Autodesk Inventor part; units mm, degrees
ref_plane "YZ Plane" through (0, 0, 0) normal (1, 0, 0) x (0, 1, 0)
ref_plane "XZ Plane" through (0, 0, 0) normal (0, 1, 0) x (-1, 0, 0)
ref_plane "XY Plane" through (0, 0, 0) normal (0, 0, 1) x (1, 0, 0)
sketch "Sketch1" plane through (0, 0, 0) normal (0, 1, 0) x (-1, 0, 0)
  line L0 (0, 0) -> (36, 0)
  line L1 (36, 0) -> (36, -24)
  line L2 (36, -24) -> (0, -24)
  line L3 (0, -24) -> (0, 0)
  dimension "d0" = 36
  dimension "d1" = 24
extrude "Extrusion1" add sketch "Sketch1" along normal blind 3
sketch "Sketch2" plane through (0, 3, 0) normal (0, 1, 0) x (1, 0, 0)
  circle A0 centre (-6, 12) radius 2.125
  point P0 (0, 0)
  dimension "d4" = 4.25
extrude "Extrusion2" cut sketch "Sketch2" against normal through all
pattern_linear "Rectangular Pattern1" count 3 spacing 12 along (-1, 0, 0) count 3 spacing 6 along (0, 0, 1) of "Extrusion2" second direction both ways yes
sketch "Sketch3" plane through (0, 0, 0) normal (1, 0, 0) x (0, 0, -1)
  line L0 (0, 0) -> (24, 0)
  line L1 (24, 0) -> (24, 3)
  line L2 (24, 3) -> (0, 3)
  line L3 (0, 3) -> (0, 0)
extrude "Extrusion3" add sketch "Sketch3" along normal blind 25
sketch "Sketch4" plane through (0, 3, 0) normal (0, 1, 0) x (1, 0, 0)
  line L0 (-36, 24) -> (25, 24)
  line L1 (25, 0) -> (22, 0)
  line L2 (22, 0) -> (22, 24)
  line L3 (22, 24) -> (25, 24)
  line L4 (25, 24) -> (25, 0)
  point P0 (0, 0)
  dimension "d15" = 3
extrude "Extrusion4" add sketch "Sketch4" along normal blind 57
sketch "Sketch5" plane through (22, 3, -24) normal (-1, 0, 0) x (0, 0, 1)
  line L0 (24, 57) -> (24, 33)
  line L1 (24, -3) -> (24, 57)
  line L2 (0, -3) -> (0, 57)
  line L3 (24, 33) -> (0, 33)
  line L4 (0, 33) -> (0, 30)
  line L5 (0, 30) -> (24, 30)
  line L6 (24, 30) -> (24, 33)
  dimension "d18" = 24
  dimension "d19" = 3
extrude "Extrusion5" add sketch "Sketch5" along normal blind 7
sketch "Sketch6" plane through (22, 36, 0) normal (0, 1, 0) x (1, 0, 0)
  line L0 (-7, 0) -> (-5, 0)
  line L1 (-5, 0) -> (-5, 2)
  line L2 (-5, 2) -> (-7, 2)
  line L3 (-7, 2) -> (-7, 0)
  line L4 (-7, 24) -> (-5, 24)
  line L5 (-5, 24) -> (-5, 22)
  line L6 (-5, 22) -> (-7, 22)
  line L7 (-7, 22) -> (-7, 24)
  point P0 (-22, 0)
  dimension "d22" = 2
  dimension "d23" = 2
  dimension "d24" = 2
  dimension "d25" = 2
extrude "Extrusion6" add sketch "Sketch6" along normal blind 24
sketch "Sketch7" plane through (25, 0, -24) normal (0, 0, -1) x (-1, 0, 0)
  line L0 (0, 60) -> (10, 60)
  line L1 (10, 60) -> (10, 33)
  line L2 (10, 33) -> (0, 33)
  line L3 (0, 33) -> (0, 60)
  point P0 (25, 0)
extrude "Extrusion7" add sketch "Sketch7" along normal blind 3
sketch "Sketch8" plane through (-36, 0, 0) normal (0, 0, 1) x (1, 0, 0)
  line L0 (51, 33) -> (61, 33)
  line L1 (61, 33) -> (61, 60)
  line L2 (61, 60) -> (51, 60)
  line L3 (51, 60) -> (51, 33)
  point P0 (36, 0)
extrude "Extrusion8" add sketch "Sketch8" along normal blind 3
sketch "Sketch9" plane through (-36, 0, 0) normal (0, 0, 1) x (1, 0, 0)
  line L0 (0, 0) -> (61, 0)
  line L1 (61, 0) -> (61, 33)
  line L2 (61, 33) -> (0, 33)
  line L3 (0, 33) -> (0, 0)
  point P0 (36, 0)
sketch "Sketch10" plane through (0, 60, 0) normal (0, 1, 0) x (1, 0, 0)
  line L0 (22, 0) -> (22, -1)
  line L1 (22, 24) -> (22, 25)
  line L2 (22, -1) -> (17, -1)
  line L3 (17, -1) -> (17, 25)
  line L4 (17, 25) -> (22, 25)
  line L5 (22, 25) -> (22, -1)
  point P0 (0, 0)
  dimension "d34" = 1
  dimension "d35" = 1
extrude "Extrusion10" cut sketch "Sketch10" against normal through all
sketch "Sketch11" plane through (-36, 0, -24) normal (0, 0, -1) x (-1, 0, 0)
  line L0 (-58, 33) -> (-58, 0)
  line L1 (-53, 0) -> (-58, 0)
  line L2 (-58, 0) -> (-58, 3)
  line L3 (-58, 3) -> (-53, 3)
  line L4 (-53, 3) -> (-53, 0)
  point P0 (-36, 0)
extrude "Extrusion11" add sketch "Sketch11" against normal blind 24
sketch "Sketch12" plane through (-36, 0, -24) normal (0, 0, -1) x (-1, 0, 0)
  line L0 (-36, 0) -> (0, 20.7846)
  line L1 (-36, 0) -> (5.5692, 0) construction
  line L2 (0, 20.7846) -> (-1.5, 23.3827)
  line L3 (-1.5, 23.3827) -> (-37.5, 2.5981)
  line L4 (-37.5, 2.5981) -> (-36, 0)
  dimension "d47" = 30
  dimension "d48" = 3
ref_plane "Work Plane1" through (0.3404, 3, 0) normal (0.2240446, 0.9745789, 0) x (0.9745789, -0.2240446, 0)
extrude "Extrusion14" add sketch "Sketch12" against normal blind 24
sketch "Sketch15" plane through (-36, 0, -24) normal (0, 0, -1) x (-1, 0, 0)
  line L0 (0, 3) -> (-30.8038, 3)
  line L1 (0, 3) -> (-30.8038, 3)
  line L2 (-30.8038, 3) -> (-36, 0)
  line L3 (-36, 0) -> (0, 0)
  line L4 (0, 0) -> (-61, 0)
  line L5 (0, 0) -> (0, 3)
extrude "Extrusion15" cut sketch "Sketch15" against normal through all
sketch "Sketch16" plane through (0.8038, 3, 0) normal (0.5, 0.8660254, 0) x (0.8660254, -0.5, 0)
  line L0 (-40.7654, 24) -> (-40.7654, 0)
  line L1 (-40.7654, 12) -> (-34.7654, 12)
  circle A0 centre (-34.7654, 12) radius 2.125
  point P0 (0.8038, 0)
  dimension "d53" = 6
  dimension "d54" = 4.25
extrude "Extrusion16" cut sketch "Sketch16" against normal through all
pattern_linear "Rectangular Pattern2" count 3 spacing 12 along (0.8660254, -0.5, 0) count 3 spacing 6 along (0, 0, 1) of "Extrusion16" second direction both ways yes
equation "\"d5\" = d4"
properties part number "PiCamWalkerMount"
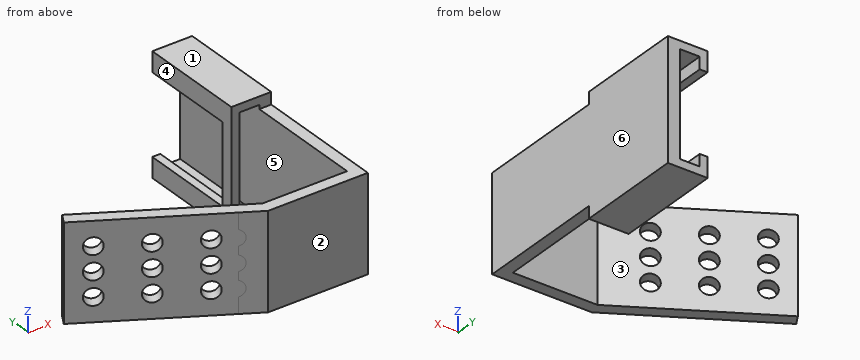
Geometry check sheet. Reference: the model listing, model coordinates, mm. Face numbers are marked on the shaded views. A direction names the side the tool comes from. Give positions to 0.01 mm unless a question says otherwise; leave off trailing zeros. Loops run counter-clockwise (first coordinate to the right, second up) from the corner with the lowest first, then second, coordinate; pieces in that order, holes last. Notation, with made-up numbers: M 55.25,62 L 96.25,62 A6 ccw 96.25,69 Z; hole C 80.5,27 d10. An arc over 180 degrees is marked long. Answer as CSV lines item,"result".
Item 1: Depth check by flat-ended pin: P1, Ø4, axis at x = 7.5, z = -22.5, coming from the -Y side; P2, Ø6, axis at y = 21.5, z = -19.5, coming from the -X side; P3, Ø6, axis at y = 17, z = -23.5, coming from the -X side; P4, Ø13.5, axis at y = 50, z = -5.5, coming from the -X side. Enter the tip coordinate at first touch or a pass-through.
Values:
P1,"stops at y = 0"
P2,"stops at x = -36"
P3,"stops at x = -34.64"
P4,"stops at x = 15"
Item 2: Cross-section at A-A on x = 20.5. Record the cut outline in (y, z).
Values:
outline,"M 0,-24 L 3,-24 L 3,0 L 0,0 Z; M 33,-27 L 60,-27 L 60,-25 L 33,-25 Z; M 33,1 L 60,1 L 60,3 L 33,3 Z"
Item 3: Release check for a two-part mould opening along Y. For the marked faces 1, 2 and 3 record: pulls with the +Y half, pulls with the -Y half, needs draft (parallel to the pull), parting line crosses it, or undercut.
Values:
face 1,"needs draft"
face 2,"pulls with the -Y half"
face 3,"pulls with the +Y half"
Item 4: Access from +Z, -Z, +X, -X, +Y, -Y to the whole of each face (thin tool, end or side, straight path). Record for the marked faces 4, 5 and 6.
Values:
face 4,"+Z, -Z, -X, +Y"
face 5,"+Y"
face 6,"+Z, -Z, +X, +Y, -Y"
Item 5: Cross-section at D-D on x = -9.5. Count the separate pieces of the cut face and the enclosed holes in it, and give its area (3 significant figures).
Values:
separate pieces,"4"
enclosed holes,"0"
area,"40.6 mm²"
Item 6: Cross-section at B-B on z = -18.75. Record the cut outline in (x, y).
Values:
outline,"M -36,20.78 L -32.53,18.78 L -31.03,21.38 L -34.5,23.38 Z; M -29.08,16.79 L -22.13,12.78 L -20.63,15.38 L -27.58,19.39 Z; M -18.69,10.79 L -11.74,6.78 L -10.24,9.38 L -17.19,13.39 Z; M -8.3,4.79 L -4.01,2.32 L 0,0 L 25,0 L 25,60 L 22,60 L 22,3 L 0.8,3 L -6.8,7.39 Z; M 15,33 L 17,33 L 17,36 L 15,36 Z"
Item 7: Cross-section at C-C on y = 26.5. Record the cut outline in (x, z), and give its area (3 significant figures).
Values:
outline,"M 22,-24 L 25,-24 L 25,0 L 22,0 Z"
area,"72.0 mm²"
Item 8: Material ranges on line 1 (X direction, y = 40, z = -1); line 2 (X direction, y = 37.5, z = -11); line 3 (X direction, y = 9, z = -6), recorded low to high.
Values:
line 1,"x = 15 to 17, 22 to 25"
line 2,"x = 22 to 25"
line 3,"x = -15.59 to -10.62, 22 to 25"
